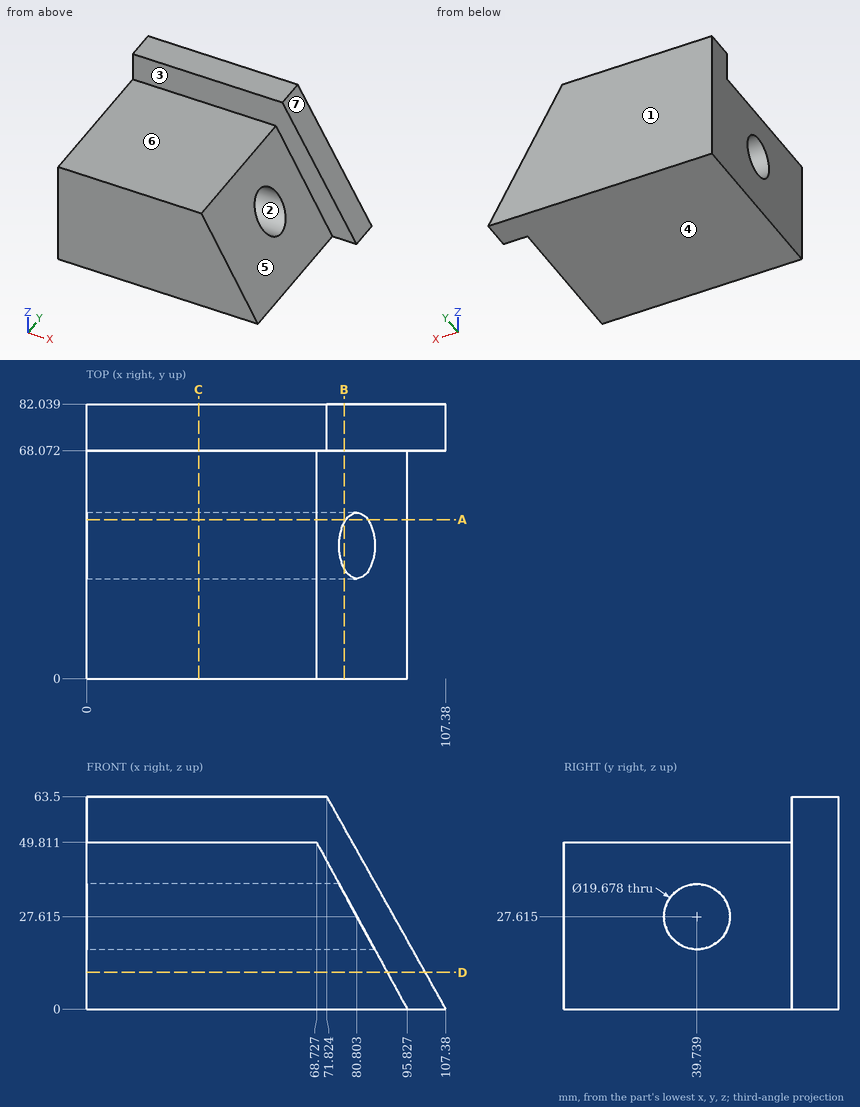
Can you work these out from the drawing? Everything is in mm from the part's minimum corner. A direction names the side the tool comes from. Coordinates: 2 decimals unless noted, no trailing zeros. Write each loop counter-clockwise with the first axis right and the second up, starting at its lowest first coordinate (ties: lowest second). Pieces come first, ordered by that corner, then holes. Notation, with made-up numbers: (71.5, -21) - (122.5, -21) arc R18 ccw to (122.5, 8) - close; hole circle Ø3 at (30, -17.5). An arc over 180 degrees is marked (long way). One line per item, written item: value.
1) I need wall thicknesses on line 1 along Y through (x, z) = (23, 27); line 2 along Z through (x, y) = (66, 40); line 3 along Z through (x, y) = (26.5, 51.5). Which ranges of each line are inside material? Lowest first, please.
Model answer:
line 1: y = 0 to 29.92, 49.56 to 82.04
line 2: z = 0 to 17.78, 37.45 to 49.81
line 3: z = 0 to 49.81
2) On a 3-axis mill with a long thin cutter (end or side, diameter ignored), from which of +Z, -Z, +X, -X, +Y, -Y can I reach the whole of each face in a straight line? I mean the marked faces 5, 6 and 7. Say none if no direction works.
Model answer:
face 5: +Z, +X, -Y
face 6: +Z, +X, -X, -Y
face 7: +Z, +X, +Y, -Y
3) I'm going to push flat-ended pins straight in: P1, Ø1, axis at y = 64.5, z = 51.5, coming from the +X side; P2, Ø12, axis at x = 41.5, z = 14.5, coming from the -Y side; P3, Ø3, axis at x = 87.5, z = 22, coming from the -Y side; P4, Ø1, axis at x = 83, y = 43.5, coming from the +Z side. Where does each tip first touch, or does it pass through?
Model answer:
P1: passes through
P2: stops at y = 0
P3: stops at y = 68.07
P4: stops at z = 18.75
4) Suppose I cut it at B-B on x = 77. Write out the boundary of the cut face in (y, z) (1 decimal).
Model answer:
outline: (0, 0) - (82, 0) - (82, 54.3) - (68.1, 54.3) - (68.1, 34.6) - (46.7, 34.6) arc R9.8 cw (long way) to (32.8, 34.6) - (0, 34.6) - close
5) Suppose I cut it at C-C on x = 33.5. Write out the boundary of the cut face in (y, z) (1 decimal).
Model answer:
outline: (0, 0) - (82, 0) - (82, 63.5) - (68.1, 63.5) - (68.1, 49.8) - (0, 49.8) - close; hole circle Ø19.7 at (39.7, 27.6)
6) Suppose I cut it at A-A on y = 47.5. Write out the boundary of the cut face in (x, z), and give its area (3 significant figures).
Model answer:
outline: (0, 0) - (95.83, 0) - (84.09, 21.57) - (0, 21.57) - close; (0, 33.66) - (77.51, 33.66) - (68.73, 49.81) - (0, 49.81) - close
area: 3,120 mm²
7) We'd pull the mould along Y, two halves only. Please class the marked faces 1, 2, 3 and 4: pulls with the +Y half, pulls with the -Y half, needs draft (parallel to the pull), parting line crosses it, or undercut.
Model answer:
face 1: pulls with the +Y half
face 2: undercut
face 3: pulls with the -Y half
face 4: needs draft
8) Suppose I cut it at D-D on z = 11. Write out the boundary of the cut face in (x, y), and give its area (3 significant figures).
Model answer:
outline: (0, 0) - (89.84, 0) - (89.84, 68.07) - (101.22, 68.07) - (101.22, 82.04) - (0, 82.04) - close
area: 7,530 mm²
